from build123d import *

# Parameters (mm, degrees)
ESQUISSE1_W             = 185
ESQUISSE1_H             = 40
BOSS_EXTRU_1_DEPTH      = 50
ESQUISSE2_R             = 15.509184
ENL_V_MAT_EXTRU_1_DEPTH = 185
CHANFREIN1_SIZE         = 6
ESQUISSE3_R             = 2
ENL_V_MAT_EXTRU_2_DEPTH = 15
ESQUISSE4_W             = 40
ESQUISSE4_H             = 10
ENL_V_MAT_EXTRU_3_DEPTH = 50


with BuildPart() as part:
    # Esquisse1 → Boss.-Extru.1 (new body)
    with BuildSketch(Plane.XY):
        with Locations((92.5, 20)):
            Rectangle(ESQUISSE1_W, ESQUISSE1_H)
    extrude(amount=BOSS_EXTRU_1_DEPTH)

    # Esquisse2 → Enlèv. mat.-Extru.1 (cut)
    with BuildSketch(Plane.ZY):
        with Locations((25, 20)):
            Circle(ESQUISSE2_R)
    extrude(amount=-ENL_V_MAT_EXTRU_1_DEPTH, mode=Mode.SUBTRACT)

    # Chanfrein1
    chanfrein1_edges = [part.edges().sort_by_distance(p)[0] for p in [
        (92.5, 40, 50),
        (92.5, 40, 0),
    ]]
    chamfer(chanfrein1_edges, length=CHANFREIN1_SIZE)

    # Esquisse3 → Enlèv. mat.-Extru.2 (cut)
    with BuildSketch(Plane.XZ):
        with Locations(Location((6, 44, 0), (0, 0, 270))):
            Circle(ESQUISSE3_R)
        with Locations(Location((6, 6, 0), (0, 0, 90))):
            Circle(ESQUISSE3_R)
        with Locations(Location((179, 6, 0), (0, 0, 270))):
            Circle(ESQUISSE3_R)
        with Locations(Location((179, 44, 0), (0, 0, 90))):
            Circle(ESQUISSE3_R)
    extrude(amount=-ENL_V_MAT_EXTRU_2_DEPTH, mode=Mode.SUBTRACT)

    # Esquisse4 → Enlèv. mat.-Extru.3 (cut)
    with BuildSketch(Plane.XY.offset(50)):
        with Locations((92.5, 35)):
            Rectangle(ESQUISSE4_W, ESQUISSE4_H)
    extrude(amount=-ENL_V_MAT_EXTRU_3_DEPTH, mode=Mode.SUBTRACT)


solid = part.part
The model under review builds one solid part; all positions refer to its coordinate system, in mm. A direction names the side the tool comes from. Give positions to 0.01 mm unless a question says otherwise; leave off trailing zeros. Loops run counter-clockwise (first coordinate to the right, second up) from the corner with the lowest first, then second, coordinate; pieces in that order, holes last. Notation, with made-up numbers: (31, -8.75) -> (48, -8.75) arc R16 cw to (48, 0.25) -> close; hole circle Ø7 at (58, 85.5). An arc over 180 degrees is marked (long way). Put each result on its own line as item: value. Start each with the question number.
1. We need section D-D on y = 23. State the section outline as (x, z) points.
2. We need section B-B on z = 25. State the section outline as (x, y) points, then the cut area to 3 significant figures.
3. Wall thickness on probe 1 along X at (y, z) = (11, 44); probe 2 along Y at (x, z) = (56.5, 25); probe 3 along X at (y, z) = (34, 39): over which ranges is each line inside the solid? List them lowest first.
4. We need section A-A on x = 6. State the section outline as (y, z) points.
5. Clearance check with flat-ended pins moving along their axes: P1, Ø1.2, axis at x = 179, z = 6, coming from the -Y side; P2, Ø6.5, axis at x = 86, z = 8, coming from the +Y side. State where each tip first meets the part, or that it passes through.
6. For faces 1 (the face through (179, 15, 44)), 2 (the face through (92, 30, 7)), 3 (the face through (36, 37, 47)), list the 3-axis set-ups (+Z, -Z, +X, -X, +Y, -Y) from which the entire face can be reached by the end or side of a thin tool; tool diameter is ignored.
7. We need section C-C on y = 13. State the section outline as (x, z) points, then the cut area to 3 significant figures.
8. Mouldability with a two-part tool opening along Y and no side actions: class faces 4 (the face through (91, 17, 0)), 5 (the face through (91.205, 6.241, 32.157)), 6 (the face through (148, 40, 25)), 7 (the face through (6, 15, 6)) as released by +Y, released by -Y, zero draft, split by the parting line, or undercut.
Determined:
1. outline: (0, 0) -> (185, 0) -> (185, 9.78) -> (0, 9.78) -> close; (0, 40.22) -> (185, 40.22) -> (185, 50) -> (0, 50) -> close
2. outline: (0, 0) -> (185, 0) -> (185, 4.49) -> (0, 4.49) -> close; (0, 35.51) -> (72.5, 35.51) -> (72.5, 40) -> (0, 40) -> close; (112.5, 35.51) -> (185, 35.51) -> (185, 40) -> (112.5, 40) -> close
2. area: 1,480 mm^2
3. probe 1: 0 to 4, 8 to 177, 181 to 185
3. probe 2: 0 to 4.49, 35.51 to 40
3. probe 3: 0 to 72.5, 112.5 to 185
4. outline: (0, 0) -> (34, 0) -> (40, 6) -> (40, 44) -> (34, 50) -> (0, 50) -> (0, 46) -> (15, 46) -> (15, 42) -> (0, 42) -> (0, 8) -> (15, 8) -> (15, 4) -> (0, 4) -> close; hole circle Ø31.02 at (20, 25)
5. P1: y = 15
5. P2: y = 30
6. face 1: -Y
6. face 2: +Z, -Z, +Y
6. face 3: +Z, +X, -X, +Y
7. outline: (0, 0) -> (185, 0) -> (185, 11.16) -> (0, 11.16) -> close; (0, 38.84) -> (185, 38.84) -> (185, 50) -> (0, 50) -> close; hole circle Ø4 at (6, 6); hole circle Ø4 at (6, 44); hole circle Ø4 at (179, 6); hole circle Ø4 at (179, 44)
7. area: 4,080 mm^2
8. face 4: zero draft
8. face 5: undercut
8. face 6: released by +Y
8. face 7: released by -Y
